Part model, mm, in its own coordinate system. A direction names the side the tool comes from. Give positions to 0.01 mm unless a question says otherwise; leave off trailing zeros. Write each loop counter-clockwise with the first axis right and the second up, starting at its lowest first coordinate (ties: lowest second). Pieces come first, ordered by that corner, then holes. Notation, with made-up numbers: M 57.25,83 L 100.25,83 A11 cw 100.25,87 Z; hole C 80,36 d6. An arc over 180 degrees is marked long. Use CSV: the item, a comma, the result in double quotes. Start each with the question number.
Item 1: Mould opens along Z. For faces 4 (the cylindrical face through (-0.07, -2.44, 0.54)), 5 (the cylindrical face through (4.754, -1.341, -3.233)), 6 (the conical face through (-4.85, 9.81, -2.18)), 7 (the flat face through (5, 7.3, -3.7)) say: released by +Z, released by -Z, zero draft, split by the parting line, or undercut.
Item 2: Cut at B-B (x = 3). List the corners of the cut face in (y, z), then the cut area to 3 significant figures.
Item 3: Drill centre lines: line 1 (Y direction, x = 4.7, z = 0); line 2 (X direction, y = 4.5, z = 0.75); line 3 (X direction, y = -3, z = 4.5). Where is each one in solid material? Low to high. Write a range as [from, to].
Item 4: Cut at A-A (x = -3.5). List the corners of the cut face in (y, z).
Item 5: Pin check, flat tips, straight feed: pin 1 (3 mm diameter, centred on x = -3, z = -5, fed in from +Y); pin 2 (1 mm diameter, centred on y = 7.5, z = 8.5, fed in from +X); pin 3 (1.5 mm diameter, centred on x = 2, z = -1.5, fed in from -Y). Stop position of each tip, or through.
Item 6: Which spindle directions (+Z, -Z, +X, -X, +Y, -Y) get a long thin tool onto all of the face, cutting with end or side? Do faces 1 (the flat face through (-4.75, 4, 4)), 2 (the cylindrical face through (4.75, 7.81, -1.73)), 3 (the flat face through (5, -2, -2)). Say none if no direction does.
from build123d import *

# Parameters (mm, degrees)
SKETCH3_R           = 8
SKETCH3_R_2         = 6
BOSS_EXTRUDE1_DEPTH = 4.5
SKETCH3_4_R         = 6
SKETCH3_4_R_2       = 5
BOSS_EXTRUDE3_DEPTH = 4.75
SKETCH3_5_R         = 5
SKETCH3_5_R_2       = 3.5
BOSS_EXTRUDE4_DEPTH = 4.5
SKETCH3_6_R         = 3.5
SKETCH3_6_R_2       = 2.5
BOSS_EXTRUDE5_DEPTH = 5


with BuildPart() as part:
    # Sketch2 → Revolve1 (revolve)
    with BuildSketch(Plane.XY, mode=Mode.PRIVATE) as revolve1_sk:
        Polygon((-5, 8), (-5, 9.9), (-2.65, 12.25), (2.65, 12.25), (5, 9.9), (5, 8), align=None)
    revolve(revolve1_sk.sketch.rotate(Axis((-45.586046512, 0, 0), (1, 0, 0)), 90), axis=Axis((-45.586046512, 0, 0), (1, 0, 0)))

    # Sketch3 → Boss-Extrude1 (add, symmetric)
    with BuildSketch(Plane(origin=(0, 0, 0), x_dir=(0, 0, -1), z_dir=(1, 0, 0))):
        with Locations(Location((0, 0, 0), (0, 0, 180))):
            Circle(SKETCH3_R)
        Circle(SKETCH3_R_2, mode=Mode.SUBTRACT)
    extrude(amount=BOSS_EXTRUDE1_DEPTH, both=True)

    # Sketch3_4 → Boss-Extrude3 (add, symmetric)
    with BuildSketch(Plane(origin=(0, 0, 0), x_dir=(0, 0, -1), z_dir=(1, 0, 0))):
        Circle(SKETCH3_4_R)
        Circle(SKETCH3_4_R_2, mode=Mode.SUBTRACT)
    extrude(amount=BOSS_EXTRUDE3_DEPTH, both=True)

    # Sketch3_5 → Boss-Extrude4 (add, symmetric)
    with BuildSketch(Plane(origin=(0, 0, 0), x_dir=(0, 0, -1), z_dir=(1, 0, 0))):
        Circle(SKETCH3_5_R)
        Circle(SKETCH3_5_R_2, mode=Mode.SUBTRACT)
    extrude(amount=BOSS_EXTRUDE4_DEPTH, both=True)

    # Sketch3_6 → Boss-Extrude5 (add, symmetric)
    with BuildSketch(Plane(origin=(0, 0, 0), x_dir=(0, 0, -1), z_dir=(1, 0, 0))):
        Circle(SKETCH3_6_R)
        Circle(SKETCH3_6_R_2, mode=Mode.SUBTRACT)
    extrude(amount=BOSS_EXTRUDE5_DEPTH, both=True)


solid = part.part
Worked answers:
1,face 4,"undercut"
1,face 5,"undercut"
1,face 6,"split by the parting line"
1,face 7,"zero draft"
2,outline,"C 0,0 d23.8; hole C 0,0 d5"
2,area,"425 mm^2"
3,line 1,"y = [-10.2, -8], [-6, -5], [-3.5, -2.5], [2.5, 3.5], [5, 6], [8, 10.2]"
3,line 2,"x = [-4.5, 4.5]"
3,line 3,"x = [-4.75, 4.75]"
4,outline,"C 0,0 d22.8; hole C 0,0 d5"
5,pin 1,"stops at y = 11.73"
5,pin 2,"stops at x = 4.06"
5,pin 3,"stops at y = -12.23"
6,face 1,"-X"
6,face 2,"+X"
6,face 3,"+Z, -Z, +X, +Y, -Y"
